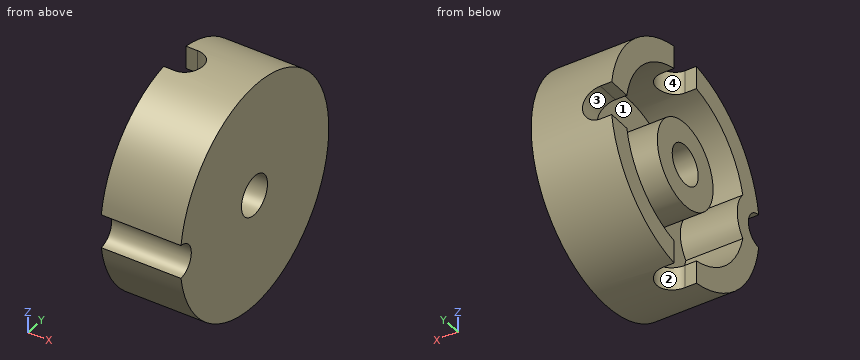
Autodesk Inventor part; units mm, degrees
ref_plane "YZ Plane" through (0, 0, 0) normal (1, 0, 0) x (0, 1, 0)
ref_plane "XY Plane" through (0, 0, 0) normal (0, 0, 1) x (1, 0, 0)
sketch "Эскиз1" plane through (0, 0, 0) normal (0, 1, 0) x (-1, 0, 0)
  line L0 (5.6588, 0) -> (-7.527, 0) construction
  line L1 (0, 0) -> (0, 1.75) construction
  line L2 (0, 1.75) -> (0, 10)
  line L3 (0, 10) -> (7, 10)
  line L4 (7, 10) -> (7, 8)
  line L5 (7, 8) -> (2, 8)
  line L6 (2, 8) -> (2, 3.75)
  line L7 (2, 3.75) -> (7, 3.75)
  line L8 (7, 3.75) -> (7, 1.75)
  line L9 (7, 1.75) -> (0, 1.75)
  dimension "d0" = 1.75
  dimension "d1" = 8.25
  dimension "d2" = 7
  dimension "d3" = 2
  dimension "d4" = 5
  dimension "d5" = 4.25
  dimension "d6" = 2
revolve "Вращение1" add sketch "Эскиз1" angle 360 about axis through (-5.6588, 0, 0) along (1, 0, 0)
ref_plane "РабПлоскость1" through (0, 10, 0) normal (0, 1, 0) x (-1, 0, 0)
sketch "Эскиз3" plane through (0, 10, 0) normal (0, 1, 0) x (-1, 0, 0)
  line L0 (7, -3.75) -> (7, 3.75) construction
  line L1 (7, 0) -> (7, 1.5) construction
  line L2 (7, 1.5) -> (6, 1.5)
  line L3 (7, 0) -> (7, -1.5) construction
  line L4 (7, -1.5) -> (6, -1.5)
  arc A0 (6, 1.5) -> (6, -1.5) centre (6, 0) ccw
  line L5 (7, 1.5) -> (7, -1.5)
  point P0 (0, 0)
  dimension "d12" = 1.5
  dimension "d13" = 1
  dimension "d14" = 1.5
  dimension "d15" = 1
extrude "Выдавливание1" cut sketch "Эскиз3" against normal blind 2.5
sketch "Эскиз4" plane through (-7, 0, 0) normal (-1, 0, 0) x (0, 0, 1)
  point P0 (0, 0)
  point P1 (0, 0)
pattern_circular "Круговой массив1" count 2 over 90 about axis through (-3.5, 0, 0) along (-1, 0, 0) of "Выдавливание1"
pattern_circular "Круговой массив2" count 2 over 90 about axis through (-3.5, 0, 0) along (1, 0, 0) of "Выдавливание1"
sketch "Эскиз5" plane through (-7, -1.5, -9.8869) normal (-1, 0, 0) x (0, 0, 1)
  line L0 (9.8869, 1.5) -> (9.8869, -10.507) construction
  arc A0 (0, 0) -> (19.7737, 0) centre (9.8869, 1.5) ccw
  arc A1 (11.3838, -8.4049) -> (8.3911, -8.3878) centre (9.8869, -8.5) ccw
  point P0 (11.3826, -8.3875)
  point P1 (8.3911, -8.3875)
  dimension "d24" = 1.5
extrude "Выдавливание2" cut sketch "Эскиз5" against normal blind 7
sketch "Эскиз7" plane through (-7, -1.5, -9.8869) normal (-1, 0, 0) x (0, 0, 1)
  circle A0 centre (9.8869, -8.5) radius 3
  point P0 (9.8869, 1.5)
  dimension "d28" = 6
extrude "Выдавливание3" add sketch "Эскиз7" against normal blind 7
sketch "Эскиз8" plane through (-7, -1.5, -9.8869) normal (-1, 0, 0) x (0, 0, 1)
  circle A0 centre (9.8869, 1.5) radius 10
  dimension "d31" = 20
extrude "Выдавливание4" cut sketch "Эскиз8" against normal blind 7 keep common part
sketch "Эскиз9" plane through (-7, -1.5, -9.8869) normal (-1, 0, 0) x (0, 0, 1)
  circle A0 centre (9.8869, 1.5) radius 10
  circle A1 centre (9.8869, -8.5) radius 1.5
  point P0 (11.3826, -8.3875)
  point P1 (8.3911, -8.3875)
  dimension "d34" = 3
extrude "Выдавливание5" cut sketch "Эскиз9" against normal blind 7 contours A1 A0 picked at (9.8869, -7.9917)
properties part number "Сердечник"
Design review of the part built by this model. Coordinates are the model's own, in mm. Face numbers are marked on the shaded views. A direction names the side the tool comes from. Coordinates: 2 decimals unless noted, no trailing zeros. Order: outer loops, then holes, each group sorted by start corner. A loop starts at its lowest first (then second) coordinate and runs counter-clockwise, first axis right, second up. Notation, with made-up numbers: (35, -9) -> (93, -9) arc R19 ccw to (93, 24) -> close; hole circle Ø3 at (56.5, -24.5). An arc over 180 degrees is marked (long way). Use one line per item in the form item = value. Start each with the question number.
(1) Add section C-C on y = 0. State the section outline as (x, z) points.
(2) Add section A-A on x = -3. State the section outline as (y, z) points, plus the area to 3 significant figures.
(3) For the marked faces 1, 2, 3 and 4, list the 3-axis set-ups (+Z, -Z, +X, -X, +Y, -Y) from which the entire face can be reached by the end or side of a thin tool; tool diameter is ignored.
(4) Add section D-D on x = -5. State the section outline as (y, z) points.
(5) Add section B-B on z = 0. State the section outline as (x, y) points.
(6) Insertion check: pin 1 (1.1 mm diameter, centred on x = -6.5, y = 9, fed in from -Z); pin 2 (3 mm diameter, centred on x = -4.5, y = -2.5, fed in from -Z); pin 3 (1.1 mm diameter, centred on x = -6.5, z = -8.5, fed in from +Y); pin 4 (6 mm diameter, centred on y = -5.5, z = -3, fed in from +X). Each pin has a flat end and moves straight along its axis. Give the tip position at first contact, or say it passes through.
(7) For probe 1 along Z at (x, y) = (-3.1, 0); probe 2 along Y at (x, z) = (-4, 0); probe 3 along X at (y, z) = (-6.5, -0.25), list the stretches that pass through material, from the lowest coordinate up.
Answer block:
q1.outline = (-7, -3.75) -> (-2, -3.75) -> (-2, -8) -> (-4.5, -8) -> (-4.5, -10) -> (0, -10) -> (0, -1.75) -> (-7, -1.75) -> close; (-7, 1.75) -> (0, 1.75) -> (0, 10) -> (-4.5, 10) -> (-4.5, 8) -> (-2, 8) -> (-2, 3.75) -> (-7, 3.75) -> close
q2.outline = (-9.89, -1.5) arc R10 ccw (long way) to (-9.89, 1.5) arc R1.5 cw to start; circle Ø7.5 at (0, 0); hole (-7.75, -1.98) arc R8 ccw (long way) to (-7.75, 1.98) arc R3 cw to start; hole circle Ø3.5 at (0, 0)
q2.area = 147 mm²
q3.face_1 = -X
q3.face_2 = -Z, -X
q3.face_3 = -X, +Y
q3.face_4 = +Z, -X
q4.outline = (-9.89, -1.5) arc R10 ccw to (-1.12, -9.94) -> (-1.12, -7.92) arc R8 cw to (-7.75, -1.98) arc R3 ccw to (-7.75, 1.98) arc R8 cw to (-1.12, 7.92) -> (-1.12, 9.94) arc R10 ccw to (-9.89, 1.5) arc R1.5 cw to start; circle Ø7.5 at (0, 0); (1.12, -9.94) arc R10 ccw to (9.94, -1.12) -> (7.92, -1.12) arc R8 cw to (1.12, -7.92) -> close; (1.12, 7.92) arc R8 cw to (7.92, 1.12) -> (9.94, 1.12) arc R10 ccw to (1.12, 9.94) -> close; hole circle Ø3.5 at (0, 0)
q5.outline = (-7, -8.5) -> (0, -8.5) -> (0, -1.75) -> (-7, -1.75) -> (-7, -3.75) -> (-2, -3.75) -> (-2, -7) -> (-7, -7) -> close; (-7, 1.75) -> (0, 1.75) -> (0, 10) -> (-4.5, 10) -> (-4.5, 8) -> (-2, 8) -> (-2, 3.75) -> (-7, 3.75) -> close
q6.pin_1 = -5.35
q6.pin_2 = -9.95
q6.pin_3 = 6.07
q6.pin_4 = 0
q7.probe_1 = -10 to -8, -3.75 to -1.75, 1.75 to 3.75, 8 to 10
q7.probe_2 = -8.5 to -7, -3.75 to -1.75, 1.75 to 3.75, 8 to 10
q7.probe_3 = -2 to 0
